The listing builds one solid part. Answer for the finished solid, in the listing's coordinates (mm). Face numbers are marked on the shaded views. A direction names the side the tool comes from. Round coordinates to 2 decimals unless told otherwise and drop trailing zeros. Write each loop counter-clockwise with the first axis right and the second up, starting at its lowest first coordinate (ties: lowest second). Pieces come first, ordered by that corner, then holes. Notation, with made-up numbers: M -40,-39 L 6,-39 A26 cw 6,-1 Z; hole C 3.25,85 d1. An arc over 180 degrees is marked long. One line per item, written item: value. Start each with the question number.
(1) Consider probe 1 along X at (y, z) = (-54, 11); probe 2 along Z at (x, y) = (25.5, -118.5); probe 3 along Y at (x, z) = (28.5, 15.5). Determine where each line is inside the solid, lowest interval first.
(2) Section A-A (y = -40) is taken. Determine the outline of the cut face in (x, z).
(3) Section D-D (x = 66.5) is taken. Determine the outline of the cut face in (y, z).
(4) Section C-C (z = 7.75) is taken. Determine the outline of the cut face in (x, y), plus the area to 3 significant figures.
(5) Given P1, Ø12, axis at x = 48.5, z = 9.5, coming from the +Y side; P2, Ø1.5, axis at x = 69, y = -53, coming from the +Z side; P3, Ø1, axis at y = -93.5, z = 21, coming from the +X side; P4, Ø1.6, axis at y = -94, z = 21, coming from the -X side, each flat-ended and moving along its own axis, determine where each tip first touches the part or whether it passes through.
(6) Section B-B (x = 34) is taken. Determine the outline of the cut face in (y, z), plus the area to 3 significant figures.
(7) For the marked faces 1 and 2, determine the directions among +Z, -Z, +X, -X, +Y, -Y from which every point of the face is accessible in a straight line to the end or side of a thin tool.
```python
from build123d import *

# Parameters (mm, degrees)
CROQUIS1_W              = 120
CROQUIS1_H              = 160
SALIENTE_EXTRUIR1_DEPTH = 20
CROQUIS2_W              = 28.149997618
CROQUIS2_H              = 37.819844128
CORTAR_EXTRUIR1_DEPTH   = 17
CHAFL_N1_SIZE           = 15
CROQUIS3_W              = 9.454961032
CROQUIS3_H              = 9.240075554
CROQUIS3_W_2            = 9.240075554
CROQUIS3_W_3            = 9.215154211
CROQUIS3_W_4            = 8.355073151
CROQUIS3_H_2            = 8.969416765
SALIENTE_EXTRUIR2_DEPTH = 2


with BuildPart() as part:
    # Croquis1 → Saliente-Extruir1 (new body)
    with BuildSketch(Plane.XY):
        with Locations((60, -80)):
            Rectangle(CROQUIS1_W, CROQUIS1_H)
    extrude(amount=SALIENTE_EXTRUIR1_DEPTH)

    # Croquis2 → Cortar-Extruir1 (cut)
    with BuildSketch(Plane.XY.offset(20)):
        with Locations((33.891414423, -55.610498247)):
            Rectangle(CROQUIS2_W, CROQUIS2_H)
    extrude(amount=-CORTAR_EXTRUIR1_DEPTH, mode=Mode.SUBTRACT)

    # Chaflán1
    chafl_n1_edges = [part.edges().sort_by_distance(p)[0] for p in [
        (33.891414423, -74.520420311, 3),
    ]]
    chamfer(chafl_n1_edges, length=CHAFL_N1_SIZE)

    # Croquis3 → Saliente-Extruir2 (add)
    with BuildSketch(Plane.XY.offset(20)):
        with Locations((64.727480516, -106.430913794)):
            Rectangle(CROQUIS3_W, CROQUIS3_H)
        with Locations((78.802479325, -106.430913794)):
            Rectangle(CROQUIS3_W_2, CROQUIS3_H)
        with Locations((91.975896748, -106.430913794)):
            Rectangle(CROQUIS3_W_3, CROQUIS3_H)
        with Locations((104.569940836, -106.430913794)):
            Rectangle(CROQUIS3_W_4, CROQUIS3_H)
        with Locations((64.727480516, -94.755549816)):
            Rectangle(CROQUIS3_W, CROQUIS3_H_2)
        with Locations((78.802479325, -94.755549816)):
            Rectangle(CROQUIS3_W_2, CROQUIS3_H_2)
        with Locations((91.975896748, -94.755549816)):
            Rectangle(CROQUIS3_W_3, CROQUIS3_H_2)
        with Locations((104.569940836, -94.755549816)):
            Rectangle(CROQUIS3_W_4, CROQUIS3_H_2)
    extrude(amount=SALIENTE_EXTRUIR2_DEPTH)


solid = part.part
```
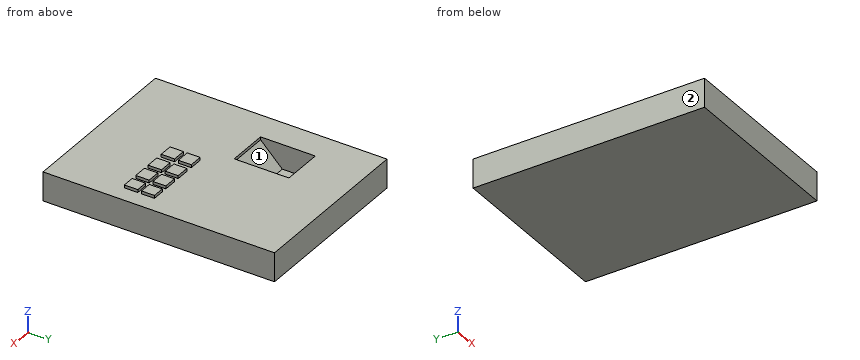
Recorded:
1. probe 1: x = 0 to 19.82, 47.97 to 120
1. probe 2: z = 0 to 20
1. probe 3: y = -160 to -72.02, -36.7 to 0
2. outline: M 0,0 L 120,0 L 120,20 L 47.97,20 L 47.97,3 L 19.82,3 L 19.82,20 L 0,20 Z
3. outline: M -160,0 L 0,0 L 0,20 L -90.27,20 L -90.27,22 L -99.24,22 L -99.24,20 L -101.81,20 L -101.81,22 L -111.05,22 L -111.05,20 L -160,20 Z
4. outline: M 0,-160 L 120,-160 L 120,0 L 0,0 Z; hole M 19.82,-64.27 L 47.97,-64.27 L 47.97,-36.7 L 19.82,-36.7 Z
4. area: 18,400 mm2
5. P1: stops at y = 0
5. P2: stops at z = 20
5. P3: stops at x = 108.75
5. P4: stops at x = 60
6. outline: M -160,0 L 0,0 L 0,20 L -36.7,20 L -36.7,3 L -59.52,3 L -74.52,18 L -74.52,20 L -160,20 Z
6. area: 2,670 mm2
7. face 1: +Z
7. face 2: +Z, -Z, -X, +Y, -Y
